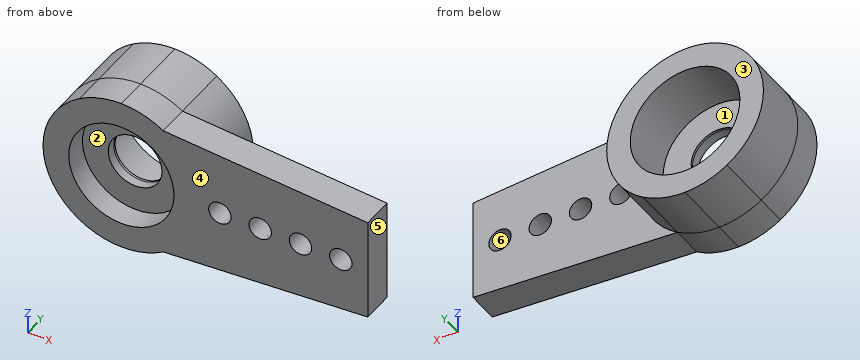
```python
from build123d import *

# Parameters (mm, degrees)
SKETCH1_R           = 0.5
BOSS_EXTRUDE1_DEPTH = 1.4
SKETCH2_R           = 2.35
CUT_EXTRUDE1_DEPTH  = 1
SKETCH3_R           = 3.5
SKETCH3_R_2         = 2.45
BOSS_EXTRUDE2_DEPTH = 2.5
SKETCH4_R           = 1.2
CUT_EXTRUDE2_DEPTH  = 20.282440198
SKETCH5_R           = 2.45
SKETCH5_R_2         = 1.2
BOSS_EXTRUDE3_DEPTH = 0.1
SKETCH6_W           = 35.735260114
SKETCH6_H           = 17.672039004
CUT_EXTRUDE4_DEPTH  = 20.513392837
CUT_EXTRUDE5_DEPTH  = 18.980545042


with BuildPart() as part:
    # Sketch1 → Boss-Extrude1 (new body)
    with BuildSketch(Plane(origin=(0, 0, 0), x_dir=(1, 0, 0), z_dir=(0, 1, 0))):
        with BuildLine():
            Line((-15.2, 2), (-2, 2.95))
            Line((-2, 2.95), (-2, 6.35))
            ThreePointArc((-2, 6.35), (0, 8.35), (2, 6.35))
            Line((2, 6.35), (2, 3.5))
            Line((2, 3.5), (11.004916923, 2.476713986))
            Line((11.004916923, 2.476713986), (11.004916923, -2.476713986))
            Line((11.004916923, -2.476713986), (2, -3.5))
            Line((2, -3.5), (2, -6.35))
            ThreePointArc((2, -6.35), (0, -8.35), (-2, -6.35))
            Line((-2, -6.35), (-2, -2.95))
            Line((-2, -2.95), (-15.2, -2))
            ThreePointArc((-15.2, -2), (-17.2, 0), (-15.2, 2))
        make_face()
        with Locations(Location((0, 6.35, 0), (0, 0, 270))):
            Circle(SKETCH1_R, mode=Mode.SUBTRACT)
        with Locations(Location((0, 4.55, 0), (0, 0, 270))):
            Circle(SKETCH1_R, mode=Mode.SUBTRACT)
        with Locations(Location((0, -4.55, 0), (0, 0, 90))):
            Circle(SKETCH1_R, mode=Mode.SUBTRACT)
        with Locations(Location((0, -6.35, 0), (0, 0, 90))):
            Circle(SKETCH1_R, mode=Mode.SUBTRACT)
        with Locations(Location((-15.2, 0, 0), (0, 0, 270))):
            Circle(SKETCH1_R, mode=Mode.SUBTRACT)
        with Locations(Location((-13.4, 0, 0), (0, 0, 270))):
            Circle(SKETCH1_R, mode=Mode.SUBTRACT)
        with Locations(Location((-11.6, 0, 0), (0, 0, 270))):
            Circle(SKETCH1_R, mode=Mode.SUBTRACT)
        with Locations(Location((-9.8, 0, 0), (0, 0, 270))):
            Circle(SKETCH1_R, mode=Mode.SUBTRACT)
        with Locations(Location((-8, 0, 0), (0, 0, 270))):
            Circle(SKETCH1_R, mode=Mode.SUBTRACT)
        with Locations(Location((-6.2, 0, 0), (0, 0, 270))):
            Circle(SKETCH1_R, mode=Mode.SUBTRACT)
        with Locations(Location((-4.4, 0, 0), (0, 0, 270))):
            Circle(SKETCH1_R, mode=Mode.SUBTRACT)
        with Locations(Location((9.8, 0, 0), (0, 0, 270))):
            Circle(SKETCH1_R, mode=Mode.SUBTRACT)
        with Locations(Location((8, 0, 0), (0, 0, 270))):
            Circle(SKETCH1_R, mode=Mode.SUBTRACT)
        with Locations(Location((6.2, 0, 0), (0, 0, 270))):
            Circle(SKETCH1_R, mode=Mode.SUBTRACT)
        with Locations(Location((4.4, 0, 0), (0, 0, 270))):
            Circle(SKETCH1_R, mode=Mode.SUBTRACT)
    extrude(amount=BOSS_EXTRUDE1_DEPTH)

    # Sketch2 → Cut-Extrude1 (cut)
    with BuildSketch(Plane.XZ):
        with Locations(Location((0, 0, 0), (0, 0, 270))):
            Circle(SKETCH2_R)
    extrude(amount=-CUT_EXTRUDE1_DEPTH, mode=Mode.SUBTRACT)

    # Sketch3 → Boss-Extrude2 (add)
    with BuildSketch(Plane(origin=(0, 1.4, 0), x_dir=(1, 0, 0), z_dir=(0, 1, 0))):
        with Locations(Location((0, 0, 0), (0, 0, 270))):
            Circle(SKETCH3_R)
        with Locations(Location((0, 0, 0), (0, 0, 270))):
            Circle(SKETCH3_R_2, mode=Mode.SUBTRACT)
    extrude(amount=BOSS_EXTRUDE2_DEPTH)

    # Sketch4 → Cut-Extrude2 (cut, through all)
    with BuildSketch(Plane(origin=(0, 1.4, 0), x_dir=(1, 0, 0), z_dir=(0, 1, 0))):
        with Locations(Location((0, 0, 0), (0, 0, 270))):
            Circle(SKETCH4_R)
    extrude(amount=-CUT_EXTRUDE2_DEPTH, mode=Mode.SUBTRACT)

    # Sketch5 → Boss-Extrude3 (add)
    with BuildSketch(Plane(origin=(0, 1.4, 0), x_dir=(1, 0, 0), z_dir=(0, 1, 0))):
        with Locations(Location((0, 0, 0), (0, 0, 270))):
            Circle(SKETCH5_R)
        with Locations(Location((0, 0, 0), (0, 0, 270))):
            Circle(SKETCH5_R_2, mode=Mode.SUBTRACT)
    extrude(amount=BOSS_EXTRUDE3_DEPTH)

    # Sketch6 → Cut-Extrude4 (cut, through all)
    with BuildSketch(Plane.XZ):
        Rectangle(SKETCH6_W, SKETCH6_H)
        with BuildLine():
            Line((-1.868584713, -2.959457918), (-15.2, -2))
            ThreePointArc((-15.2, -2), (-17.2, 0), (-15.2, 2))
            Line((-15.2, 2), (-1.868584713, 2.959457918))
            ThreePointArc((-1.868584713, 2.959457918), (0, 3.5), (1.868584713, 2.959457918))
            Line((1.868584713, 2.959457918), (15.2, 2))
            ThreePointArc((15.2, 2), (17.2, 0), (15.2, -2))
            Line((15.2, -2), (1.868584713, -2.959457918))
            ThreePointArc((1.868584713, -2.959457918), (0, -3.5), (-1.868584713, -2.959457918))
        make_face(mode=Mode.SUBTRACT)
    extrude(amount=-CUT_EXTRUDE4_DEPTH, mode=Mode.SUBTRACT)

    # Sketch7 → Cut-Extrude5 (cut, through all)
    with BuildSketch(Plane.XZ):
        with BuildLine():
            Line((0, 3.5), (-17.731768104, 3.5))
            Line((-17.731768104, 3.5), (-17.731768104, -3.5))
            Line((-17.731768104, -3.5), (0, -3.5))
            ThreePointArc((0, -3.5), (-3.5, 0), (0, 3.5))
        make_face()
    extrude(amount=-CUT_EXTRUDE5_DEPTH, mode=Mode.SUBTRACT)


solid = part.part
```
Geometry check sheet. Reference: the model listing, model coordinates, mm. Face numbers are marked on the shaded views. A direction names the side the tool comes from. Give positions to 0.01 mm unless a question says otherwise; leave off trailing zeros. Order: outer loops, then holes, each group sorted by start corner. A loop starts at its lowest first (then second) coordinate and runs counter-clockwise, first axis right, second up. Notation, with made-up numbers: (24, -6.75) - (78, -6.75) arc R9 cw to (78, 5.25) - close; hole circle Ø6 at (-11.75, 57). An arc over 180 degrees is marked (long way). Answer in a Markdown table with one row per item. Add a question column.
Q1. Gauge pin test, flat ends, axial feed: pin 1 (3 mm diameter, centred on x = 0, z = 0, fed in from -Y); pin 2 (3 mm diameter, centred on x = 8.5, z = 1, fed in from +Y); pin 3 (2 mm diameter, centred on x = 8, z = 2.5, fed in from -Y). Record the tip position at first contact, or that the pin passes through.
Q2. Material ranges on probe 1 along X at (y, z) = (1.1, 0); probe 2 along X at (y, z) = (0.9, 0); probe 3 along Y at (x, z) = (0.75, 1.5), recorded low to high. Write a range as from..to.
Q3. Cross-section at D-D, the plane y = 1.95. Enter the section's corners in (x, z).
Q4. Cross-section at A-A, the plane z = 0. Count the separate pieces of the cut face and the enclosed holes in it, then the cut area to 3 significant figures.
Q5. Tool access check on the marked faces 1, 2 and 3. Record the directions out of +Z, -Z, +X, -X, +Y, -Y that give a thin tool (end or side, any length) a straight path to the whole face; none if there is none.
Q6. Mould release check, pull along X, two halves, no side actions. Record for the marked faces 4, 5 and 6: pulls with the +X half, pulls with the -X half, needs draft (parallel to the pull), parting line crosses it, or undercut.
Q7. Cross-section at C-C, the plane y = 0.2. Enter the section's corners in (x, z), then the cut area to 4 significant figures.
Q8. Cross-section at B-B, the plane x = 4.4. Enter the section's corners in (y, z).
Check values:
| question | item | result |
|---|---|---|
| 1 | pin 1 | stops at y = 1 |
| 1 | pin 2 | stops at y = 1.4 |
| 1 | pin 3 | stops at y = 0 |
| 2 | probe 1 | x = -3.5..-1.2, 1.2..3.9, 4.9..5.7, 6.7..7.5, 8.5..9.3, 10.3..11 |
| 2 | probe 2 | x = -3.5..-2.35, 2.35..3.9, 4.9..5.7, 6.7..7.5, 8.5..9.3, 10.3..11 |
| 2 | probe 3 | y = 1..1.5 |
| 3 | outline | circle Ø7 at (0, 0); hole circle Ø4.9 at (0, 0) |
| 4 | separate pieces | 6 |
| 4 | enclosed holes | 0 |
| 4 | area | 14.5 mm^2 |
| 5 | face 1 | +Y |
| 5 | face 2 | -Y |
| 5 | face 3 | +Z, -Z, +X, -X, +Y |
| 6 | face 4 | needs draft |
| 6 | face 5 | pulls with the +X half |
| 6 | face 6 | undercut |
| 7 | outline | (1.87, -2.96) - (11, -2.3) - (11, 2.3) - (1.87, 2.96) arc R3.5 ccw (long way) to start; hole circle Ø4.7 at (0, 0); hole circle Ø1 at (4.4, 0); hole circle Ø1 at (6.2, 0); hole circle Ø1 at (8, 0); hole circle Ø1 at (9.8, 0) |
| 7 | area | 59.25 mm^2 |
| 8 | outline | (0, -2.78) - (1.4, -2.78) - (1.4, -0.5) - (0, -0.5) - close; (0, 0.5) - (1.4, 0.5) - (1.4, 2.78) - (0, 2.78) - close |
